Can you work these out from the model? Positions are in its coordinate system, mm. Give positions to 0.01 mm unless a question says otherwise; leave off trailing zeros. Loops run counter-clockwise (first coordinate to the right, second up) from the corner with the lowest first, then second, coordinate; pieces in that order, holes last.
from build123d import *

# Parameters (mm, degrees)
BOSS_EXTRUDE1_DEPTH             = 12.7
CUT_EXTRUDE1_DEPTH              = 12.7
LPATTERN1_COUNT                 = 7
LPATTERN1_PITCH                 = 46.99
CUT_EXTRUDE2_DEPTH              = 12.7
LPATTERN2_COUNT                 = 8
LPATTERN2_PITCH                 = 46.99
BOSS_EXTRUDE3_DEPTH             = 12.7
SKETCH14_R                      = 3.175
CUT_EXTRUDE5_DEPTH              = 577.697477019
SKETCH15_W                      = 50.8
SKETCH15_H                      = 15.875
CUT_EXTRUDE6_DEPTH              = 577.697477019
SKETCH16_W                      = 3.175
SKETCH16_H                      = 22.225
CUT_EXTRUDE7_DEPTH              = 44.45
CUT_EXTRUDE8_DEPTH              = 10.16
SKETCH18_W                      = 31.75
SKETCH18_H                      = 15.875
CUT_EXTRUDE9_DEPTH              = 2.54
F_1_8_0_125_DIAMETER_HOLE1_D    = 3.175
BOSS_EXTRUDE4_DEPTH             = 12.7
F_1_4_0_25_DIAMETER_HOLE1_D     = 6.35
F_1_4_0_25_DIAMETER_HOLE2_D     = 6.35
F_1_4_0_25_DIAMETER_HOLE2_DEPTH = 3.175
F_1_4_0_25_DIAMETER_HOLE2_TIP   = 1.907732465
CUT_EXTRUDE10_DEPTH             = 12.7
SKETCH28_R                      = 6.35
BOSS_EXTRUDE5_DEPTH             = 12.7
CUT_EXTRUDE11_DEPTH             = 12.7
FILLET1_R                       = 12.7
BOSS_EXTRUDE7_START             = -12.7
SKETCH30_R                      = 3.175
BOSS_EXTRUDE7_DEPTH             = 12.7
SKETCH31_R                      = 9.525
CUT_EXTRUDE12_DEPTH             = 12.7
FILLET2_R                       = 2.54
FILLET5_R                       = 2.54


with BuildPart() as part:
    # Sketch1 → Boss-Extrude1 (new body)
    with BuildSketch(Plane.XY):
        with BuildLine():
            Line((2.54, 0), (568.96, 0))
            ThreePointArc((568.96, 0), (570.756051224, 0.743948776), (571.5, 2.54))
            Line((571.5, 2.54), (571.5, 22.86))
            ThreePointArc((571.5, 22.86), (570.756051224, 24.656051224), (568.96, 25.4))
            Line((568.96, 25.4), (2.54, 25.4))
            Line((2.54, 25.4), (0, 25.4))
            Line((0, 25.4), (0, 22.86))
            Line((0, 22.86), (0, 2.54))
            Line((0, 2.54), (0, 0))
            Line((0, 0), (2.54, 0))
        make_face()
    extrude(amount=BOSS_EXTRUDE1_DEPTH)

    # Sketch2 → Cut-Extrude1 (cut)
    with BuildSketch(Plane.XY):
        with BuildLine():
            Line((173.246051224, 3.175), (205.213948776, 3.175))
            ThreePointArc((205.213948776, 3.175), (206.387275782, 3.958992041), (206.111974388, 5.343025612))
            Line((206.111974388, 5.343025612), (190.128025612, 21.326974388))
            ThreePointArc((190.128025612, 21.326974388), (189.23, 21.698948776), (188.331974388, 21.326974388))
            Line((188.331974388, 21.326974388), (172.348025612, 5.343025612))
            ThreePointArc((172.348025612, 5.343025612), (172.072724218, 3.958992041), (173.246051224, 3.175))
        make_face()
    cut_extrude1 = extrude(amount=CUT_EXTRUDE1_DEPTH, mode=Mode.SUBTRACT)

    # LPattern1: Cut-Extrude1 ×7, 1 skipped
    with Locations(*[(i * LPATTERN1_PITCH, 0, 0) for i in range(1, LPATTERN1_COUNT) if i not in (3,)]):
        add(cut_extrude1, mode=Mode.SUBTRACT)

    # Sketch3 → Cut-Extrude2 (cut)
    with BuildSketch(Plane.XY):
        with BuildLine():
            Line((149.751051224, 22.225), (181.718948776, 22.225))
            ThreePointArc((181.718948776, 22.225), (182.892275782, 21.441007959), (182.616974388, 20.056974388))
            Line((182.616974388, 20.056974388), (166.633025612, 4.073025612))
            ThreePointArc((166.633025612, 4.073025612), (165.735, 3.701051224), (164.836974388, 4.073025612))
            Line((164.836974388, 4.073025612), (148.853025612, 20.056974388))
            ThreePointArc((148.853025612, 20.056974388), (148.577724218, 21.441007959), (149.751051224, 22.225))
        make_face()
    cut_extrude2 = extrude(amount=CUT_EXTRUDE2_DEPTH, mode=Mode.SUBTRACT)

    # LPattern2: Cut-Extrude2 ×8
    with Locations(*[(i * LPATTERN2_PITCH, 0, 0) for i in range(1, LPATTERN2_COUNT)]):
        add(cut_extrude2, mode=Mode.SUBTRACT)

    # Sketch8 → Boss-Extrude3 (add)
    with BuildSketch(Plane.XY):
        Polygon((92.075, 0), (-9.525, -76.2), (-15.24, -68.58), (76.2, 0), align=None)
    extrude(amount=BOSS_EXTRUDE3_DEPTH)

    # Sketch14 → Cut-Extrude5 (cut, through all)
    with BuildSketch(Plane(origin=(0, 0, 0), x_dir=(-1, 0, 0), z_dir=(0, 0, -1))):
        with Locations((-560.3875, 12.7)):
            Circle(SKETCH14_R)
    extrude(amount=-CUT_EXTRUDE5_DEPTH, mode=Mode.SUBTRACT)

    # Sketch15 → Cut-Extrude6 (cut, through all)
    with BuildSketch(Plane.XY.offset(12.7)):
        with Locations((25.4, 12.7)):
            Rectangle(SKETCH15_W, SKETCH15_H)
    extrude(amount=-CUT_EXTRUDE6_DEPTH, mode=Mode.SUBTRACT)

    # Sketch16 → Cut-Extrude7 (cut)
    with BuildSketch(Plane.ZY):
        with Locations((7.9375, 12.7)):
            Rectangle(SKETCH16_W, SKETCH16_H)
    extrude(amount=-CUT_EXTRUDE7_DEPTH, mode=Mode.SUBTRACT)

    # Sketch17 → Cut-Extrude8 (cut)
    with BuildSketch(Plane.XY):
        Polygon((50.8, 20.6375), (54.61, 20.6375), (55.88, 22.2885), (71.12, 22.2885), (71.12, 20.6375), (107.95, 20.6375), (107.95, 4.7625), (71.12, 4.7625), (71.12, 3.1115), (55.88, 3.1115), (54.61, 4.7625), (50.8, 4.7625), align=None)
    extrude(amount=CUT_EXTRUDE8_DEPTH, mode=Mode.SUBTRACT)

    # Sketch18 → Cut-Extrude9 (cut)
    with BuildSketch(Plane(origin=(0, 0, 10.16), x_dir=(-1, 0, 0), z_dir=(0, 0, -1))):
        with Locations((-92.075, 12.7)):
            Rectangle(SKETCH18_W, SKETCH18_H)
    extrude(amount=-CUT_EXTRUDE9_DEPTH, mode=Mode.SUBTRACT)

    # 1/8 (0.125) Diameter Hole1 (through all)
    with Locations(Plane(origin=(0, 0, 10.16), x_dir=(-1, 0, 0), z_dir=(0, 0, -1))):
        with Locations((-64.77, 19.1135), (-64.77, 6.2865)):
            Hole(F_1_8_0_125_DIAMETER_HOLE1_D / 2)

    # Sketch21 → Boss-Extrude4 (add)
    with BuildSketch(Plane(origin=(0, 0, 0), x_dir=(-1, 0, 0), z_dir=(0, 0, -1))):
        with BuildLine():
            Line((-76.2, 0), (-69.85, 0))
            ThreePointArc((-69.85, 0), (-71.419048922, -1.593650359), (-71.12, -3.81))
            Line((-71.12, -3.81), (-76.2, 0))
        make_face()
    extrude(amount=-BOSS_EXTRUDE4_DEPTH)

    # 1/4 (0.25) Diameter Hole1 (through all)
    with Locations(Plane.XY.offset(12.7)):
        with Locations((133.35, 12.7), (330.2, 12.7), (527.05, 12.7)):
            Hole(F_1_4_0_25_DIAMETER_HOLE1_D / 2)

    # 1/4 (0.25) Diameter Hole2
    with Locations(Plane(origin=(0, 25.4, 0), x_dir=(1, 0, 0), z_dir=(0, 1, 0))):
        with Locations((212.616051224, -6.35), (259.606051224, -6.35)):
            Hole(F_1_4_0_25_DIAMETER_HOLE2_D / 2, depth=F_1_4_0_25_DIAMETER_HOLE2_DEPTH)
            with Locations((0, 0, -(F_1_4_0_25_DIAMETER_HOLE2_DEPTH + F_1_4_0_25_DIAMETER_HOLE2_TIP / 2))):  # 118° drill point
                Cone(0, F_1_4_0_25_DIAMETER_HOLE2_D / 2, F_1_4_0_25_DIAMETER_HOLE2_TIP, mode=Mode.SUBTRACT)

    # Sketch26 → Cut-Extrude10 (cut)
    with BuildSketch(Plane.XY.offset(12.7)):
        Polygon((-9.525, -76.2), (1.651, -67.818), (-0.254, -65.278), (-11.43, -73.66), align=None)
    extrude(amount=-CUT_EXTRUDE10_DEPTH, mode=Mode.SUBTRACT)

    # Sketch28 → Boss-Extrude5 (add)
    with BuildSketch(Plane.XY.offset(12.7)):
        Polygon((1.651, -67.818), (13.081, -83.058), (33.401, -67.818), (30.769818102, -45.978886423), align=None)
        with Locations((16.6878, -66.7004)):
            Circle(SKETCH28_R, mode=Mode.SUBTRACT)
    extrude(amount=-BOSS_EXTRUDE5_DEPTH)

    # Sketch29 → Cut-Extrude11 (cut)
    with BuildSketch(Plane.XY.offset(12.7)):
        Polygon((-15.24, -68.58), (-11.43, -73.66), (-0.254, -65.278), (-4.064, -60.198), align=None)
    extrude(amount=-CUT_EXTRUDE11_DEPTH, mode=Mode.SUBTRACT)

    # Fillet1
    fillet1_edges = [part.edges().sort_by_distance(p)[0] for p in [
        (30.769818102, -45.978886423, 6.35),
        (33.401, -67.818, 6.35),
        (13.081, -83.058, 6.35),
        (-4.064, -60.198, 6.35),
    ]]
    fillet(fillet1_edges, radius=FILLET1_R)

    # Sketch30 → Boss-Extrude7 (add)
    with BuildSketch(Plane.XY.offset(12.7).offset(BOSS_EXTRUDE7_START)):
        Polygon((578.262851122, 12.7), (578.262851122, 31.75), (542.702851122, 31.75), (542.702851122, 25.4), (542.702851122, 0), (542.702851122, -6.35), (578.262851122, -6.35), align=None)
        with Locations(Location((560.3875, 12.7, 0), (0, 0, 180))):
            Circle(SKETCH30_R, mode=Mode.SUBTRACT)
    extrude(amount=BOSS_EXTRUDE7_DEPTH)

    # Sketch31 → Cut-Extrude12 (cut)
    with BuildSketch(Plane.XY.offset(12.7)):
        with Locations((560.3875, 12.7)):
            Circle(SKETCH31_R)
    extrude(amount=-CUT_EXTRUDE12_DEPTH, mode=Mode.SUBTRACT)

    # Fillet2
    fillet2_edges = [part.edges().sort_by_distance(p)[0] for p in [
        (578.262851122, 31.75, 6.35),
        (578.262851122, -6.35, 6.35),
    ]]
    fillet(fillet2_edges, radius=FILLET2_R)

    # Fillet5
    fillet5_edges = [part.edges().sort_by_distance(p)[0] for p in [
        (542.702851122, 25.4, 6.35),
        (542.702851122, -6.35, 6.35),
        (542.702851122, 31.75, 6.35),
        (542.702851122, 0, 6.35),
    ]]
    fillet(fillet5_edges, radius=FILLET5_R)


solid = part.part
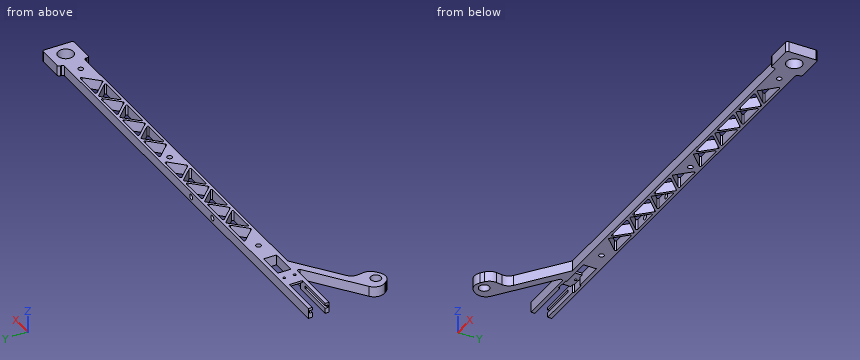
(1) Please list where these lines run through material, in increasing order: probe 1 along X at (y, z) = (25, 6.5); probe 2 along Y at (x, z) = (101.5, 11.75); probe 3 along Y at (x, z) = (457.5, 7) (3 decimals).
Returned:
probe 1: x = 0 to 209.44, 215.79 to 256.43, 262.78 to 578.26
probe 2: y = 0 to 4.76, 20.64 to 25.4
probe 3: y = 0 to 3.175, 8.555 to 13, 22.225 to 25.4
(2) Suppose I cut it at A-A on y = -13. List the corners of the cut face in (x, z) for me, plus the area to 3 significant figures.
Returned:
outline: (58.87, 0) - (74.74, 0) - (74.74, 12.7) - (58.87, 12.7) - close
area: 202 mm2
(3) Will these pins go through, and if not, where does the flat tip stop? P1, Ø6.5, axis at x = 207.5, z = 8, coming from the -Y side; P2, Ø6.5, axis at x = 381, z = 8.5, coming from the +Y side; P3, Ø1, axis at y = 22, z = 8.5, coming from the -X side.
Returned:
P1: stops at y = 0
P2: stops at y = 25.4
P3: stops at x = 44.45
